```python
from build123d import *

# Parameters (mm, degrees)
F1_R     = 1.9431
F2_DEPTH = 3.0226
F1_R_2   = 2.2987
F3_DEPTH = 6.35
F5_D     = 1.778


with BuildPart() as f2:
    # F1 (on Top) → F2 (new body)
    with BuildSketch(Plane.XY):
        Circle(F1_R)
    extrude(amount=F2_DEPTH)

    # F1 (on Top) → F3 (join)
    with BuildSketch(Plane.XY):
        Circle(F1_R_2)
        Circle(F1_R, mode=Mode.SUBTRACT)
        Circle(F1_R)
    extrude(amount=-F3_DEPTH)

    # F5 (through all)
    with Locations(Plane(origin=(0, 0, -6.35), x_dir=(1, 0, 0), z_dir=(0, 0, -1))):
        with Locations((0, 0)):
            Hole(F5_D / 2)


solid = f2.part
```
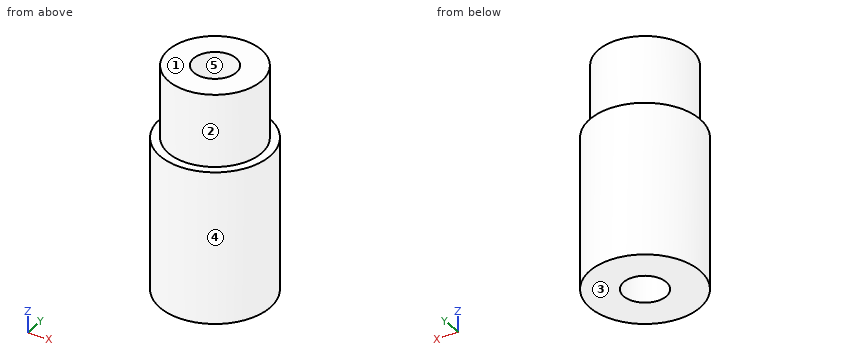
The model under review builds one solid part; all positions refer to its coordinate system, in mm. Face numbers are marked on the shaded views. A direction names the side the tool comes from. Round coordinates to 2 decimals unless told otherwise and drop trailing zeros. Loops run counter-clockwise (first coordinate to the right, second up) from the corner with the lowest first, then second, coordinate; pieces in that order, holes last. Notation, with made-up numbers: (-3.5, 26.25) -> (26.5, 26.25) arc R26 cw to (26.5, 52.25) -> close; hole circle Ø2 at (88.25, 38). An arc over 180 degrees is marked (long way). Answer as a JSON object with one key per item and string values. Group by question number.
1) We need section C-C on z = 0.5. Write out the cut boundary in (x, y), then the cut area to 3 significant figures.
2) For pin 1 Ø1.5 at (x, z) = (-1.5, -1) entering from +Y; pin 2 Ø1.5 at (y, z) = (-1, 1.5) entering from +X; pin 3 Ø2 at (y, z) = (-1.5, 0) entering from +X; pin 4 Ø1.5 at (x, z) = (0.5, -3) entering from +Y, all flat-tipped, find the tip position at first contact; note any pin that passes through.
3) For the marked faces 1 and 2, list the 3-axis set-ups (+Z, -Z, +X, -X, +Y, -Y) from which the entire face can be reached by the end or side of a thin tool; tool diameter is ignored.
4) We need section A-A on y = 0. Write out the cut boundary in (x, z), then the cut area to 3 significant figures.
5) We need section D-D on y = -1.1. Write out the cut boundary in (x, z), then the cut area to 3 significant figures.
6) For line 1 (Y direction, x = 0, z = -3.75); line 2 (Y direction, x = 0, z = 0.25), list the stretches that pass through material, from the lowest coordinate up. Write a range as [from, to].
7) Mouldability with a two-part tool opening along Y and no side actions: class the marked faces 3, 4 and 5 as released by +Y, released by -Y, zero draft, split by the parting line, or undercut.
Result set:
{
 "1": {"outline": "circle Ø3.89 at (0, 0); hole circle Ø1.78 at (0, 0)", "area": "9.38 mm²"},
 "2": {"pin 1": "y = 2.17", "pin 2": "x = 1.93", "pin 3": "x = 2.24", "pin 4": "y = 2.3"},
 "3": {"face 1": "+Z, +X, -X, +Y, -Y", "face 2": "+Z"},
 "4": {"outline": "(-2.3, -6.35) -> (-0.89, -6.35) -> (-0.89, 3.02) -> (-1.94, 3.02) -> (-1.94, 0) -> (-2.3, 0) -> close; (0.89, -6.35) -> (2.3, -6.35) -> (2.3, 0) -> (1.94, 0) -> (1.94, 3.02) -> (0.89, 3.02) -> close", "area": "24.3 mm²"},
 "5": {"outline": "(-2.02, -6.35) -> (2.02, -6.35) -> (2.02, 0) -> (1.6, 0) -> (1.6, 3.02) -> (-1.6, 3.02) -> (-1.6, 0) -> (-2.02, 0) -> close", "area": "35.3 mm²"},
 "6": {"line 1": "[-2.3, -0.89], [0.89, 2.3]", "line 2": "[-1.94, -0.89], [0.89, 1.94]"},
 "7": {"face 3": "zero draft", "face 4": "split by the parting line", "face 5": "undercut"}
}
